Could you check a few things on this model? Use its own coordinates, in mm. Coordinates: 2 decimals unless noted, no trailing zeros. Order: outer loops, then holes, each group sorted by start corner. A loop starts at its lowest first (then second) coordinate and runs counter-clockwise, first axis right, second up. Notation, with made-up numbers: (77, -1) - (128, -1) arc R21 cw to (128, 25) - close; hole circle Ø8 at (-18.5, -24.75). An arc over 180 degrees is marked (long way). One line per item, written item: value.
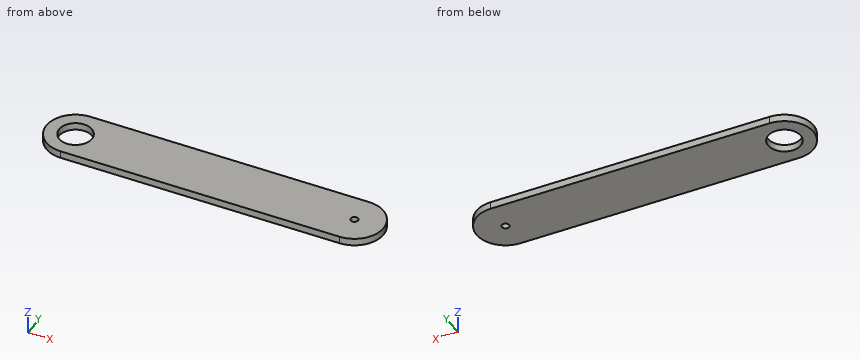
Autodesk Inventor part; units mm, degrees
ref_plane "YZ Plane" through (0, 0, 0) normal (1, 0, 0) x (0, 1, 0)
ref_plane "XZ Plane" through (0, 0, 0) normal (0, 1, 0) x (-1, 0, 0)
ref_plane "XY Plane" through (0, 0, 0) normal (0, 0, 1) x (1, 0, 0)
sketch "Sketch1" plane through (0, 0, 0) normal (0, 0, 1) x (1, 0, 0)
  circle A0 centre (0, 0) radius 14.2875
  circle A1 centre (244.475, 0) radius 3.175
  line L0 (0, 0) -> (244.475, 0) construction
  line L1 (0, 0) -> (244.475, 0) construction
  line L2 (0, -25.4) -> (244.475, -25.4)
  line L3 (244.475, 25.4) -> (0, 25.4)
  arc A2 (0, 25.4) -> (0, -25.4) centre (0, 0) ccw
  arc A3 (244.475, -25.4) -> (244.475, 25.4) centre (244.475, 0) ccw
  point P0 (122.2375, 0)
  dimension "d0" = 28.575
  dimension "d1" = 244.475
  dimension "d2" = 50.8
  dimension "d3" = 6.35
extrude "Extrusion1" add sketch "Sketch1" along normal blind 6.35
properties part number "GP4-004" material "Aluminum 6061"
Item 1: If I drill on probe 1 along X at (y, z) = (-1.5, 0.5); probe 2 along Y at (x, z) = (0, 3.25); probe 3 along X at (y, z) = (1, 5.75), over which ranges is the centre line in solid material (lowest first)?
Conclusion:
probe 1: -25.36 to -14.21, 14.21 to 241.68, 247.27 to 269.83
probe 2: -25.4 to -14.29, 14.29 to 25.4
probe 3: -25.38 to -14.25, 14.25 to 241.46, 247.49 to 269.86
Item 2: I want a section at A-A on y = 0. Give the number of separate pieces and of enclosed holes in the cut face, then the cut area to 3 significant figures.
Conclusion:
separate pieces: 3
enclosed holes: 0
area: 1,650 mm²
Item 3: I'm going to push a flat-ended pin straight in: pin 1 Ø6 at (x, y) = (148.5, 0.5) entering from -Z. Where does the tip first touch, or does it pass through?
Conclusion:
pin 1: z = 0
Item 4: I want a section at B-B on y = -11. Please give me the cut outline in (x, z).
Conclusion:
outline: (-22.89, 0) - (-9.12, 0) - (-9.12, 6.35) - (-22.89, 6.35) - close; (9.12, 0) - (267.37, 0) - (267.37, 6.35) - (9.12, 6.35) - close
